Autodesk Inventor part; units mm, degrees
ref_plane "YZ Plane" through (0, 0, 0) normal (1, 0, 0) x (0, 1, 0)
ref_plane "XZ Plane" through (0, 0, 0) normal (0, 1, 0) x (-1, 0, 0)
ref_plane "XY Plane" through (0, 0, 0) normal (0, 0, 1) x (1, 0, 0)
sketch "Skizze1" plane through (0, 0, 0) normal (0, 1, 0) x (-1, 0, 0)
  line L0 (5, 18.5) -> (-5, 18.5)
  line L1 (-5, 18.5) -> (-5, -18.5)
  line L2 (-5, -18.5) -> (5, -18.5)
  line L3 (5, -18.5) -> (5, 18.5)
  line L4 (5, 18.5) -> (-5, -18.5) construction
  line L5 (-5, 18.5) -> (5, -18.5) construction
  circle A0 centre (0, -4.75) radius 13.75 construction
  arc A1 (-5, -17.5587) -> (5, -17.5587) centre (0, -4.75) ccw
  arc A2 (5, 8.0587) -> (-5, 8.0587) centre (0, -4.75) ccw
  line L6 (0, -18.5) -> (0, 9) construction
  circle A3 centre (0, -13.75) radius 1.5
  circle A4 centre (0, 4.25) radius 1.5
  line L7 (-5, -4.75) -> (5, -4.75) construction
  circle A5 centre (0, -13.75) radius 4 construction
  circle A6 centre (0, 4.25) radius 4 construction
  circle A7 centre (0, -4.75) radius 2.75
  point P0 (0, 0)
  point P1 (0, 0)
  dimension "d2" = 37
  dimension "d3" = 10
  dimension "d4" = 27.5
  dimension "d18" = 3
  dimension "d20" = 18
  dimension "d23" = 8
  dimension "d24" = 8
  dimension "d25" = 5.5
extrude "Extrusion1" add sketch "Skizze1" along normal blind 22 contours L3 A2 L1 L0 | L3 A1 L1 A2 | A3 | A4
sketch "Skizze2" plane through (0, 0, 0) normal (1, 0, 0) x (0, 1, 0)
  line L0 (0, -18.5) -> (0, -7.5)
  line L1 (0, 18.5) -> (22, 18.5)
  line L2 (22, -7.5) -> (22, -18.5)
  line L3 (7, -18.5) -> (22, -10.5244)
  line L4 (22, -18.5) -> (0, -18.5)
  line L5 (22, -10.5244) -> (22, -18.5)
  line L6 (22, -18.5) -> (7, -18.5)
  line L7 (0, -7.5) -> (22, -7.5)
  line L8 (22, 18.5) -> (22, -2)
  line L9 (22, -2) -> (0, -2)
  line L10 (0, -2) -> (0, 18.5)
  dimension "d14" = 62
  dimension "d15" = 7
extrude "Extrusion5" cut sketch "Skizze2" along normal through all both and the other way through all contours L3 L2 L4
extrude "Extrusion3" cut sketch "Skizze1" along normal blind 5 contours L3 A1 L1 A2 | L3 L2 A1 | A1 L2 L1 | A3 | A4 | A7
extrude "Extrusion6" cut sketch "Skizze1" along normal blind 11 contours A3 | A4
fillet "Rundung1" radius 1 9 edges at (5, 22, 3.9878) (-5, 22, 3.9878) (0, 22, -10.5244) (5, 15.3852, -14.0415) (5, 6.8852, -17.5587) (-5, 6.8852, -17.5587) (-5, 15.3852, -14.0415) (-5, 11, 18.5) (5, 11, 18.5)
properties part number "Schalter_Knauf"
Input: part model. Units: mm. Frame: model coordinates. A direction names the side the tool comes from. Coordinates: 2 decimals unless noted, no trailing zeros. Loops run counter-clockwise (first coordinate to the right, second up) from the corner with the lowest first, then second, coordinate; pieces in that order, holes last.
Q1. Section B-B, the plane z = 4.25. Return the cut outline in (x, y).
Results are:
outline: (-5, 5) - (-1.5, 5) - (-1.5, 11) - (1.5, 11) - (1.5, 5) - (5, 5) - (5, 21) arc R1 ccw to (4, 22) - (-4, 22) arc R1 ccw to (-5, 21) - close
Q2. Contact query for flat-ended pins moving along their axis: pin 1 (3.5 mm diameter, centred on x = 0, z = -13.75, fed in from -Y); pin 2 (6 mm diameter, centred on x = -3, y = 9, fed in from -Z); pin 3 (1.5 mm diameter, centred on x = -0.5, z = 4.5, fed in from -Y); pin 4 (4.5 mm diameter, centred on x = 0, z = -4.75, fed in from +Y). Output: stop coordinate, or through.
Results are:
pin 1: stops at y = 5
pin 2: stops at z = -18.48
pin 3: stops at y = 11
pin 4: passes through
Q3. Set-up query: faces 1 (the flat face through (0, 11, -14)), 2 (the flat face through (5, 10, 4)), 3 (the cylindrical face through (0, 2, 9)). Return all of +Z, -Z, +X, -X, +Y, -Y with unobstructed straight access to the full face (end or side cutting, diameter ignored); none if empty.
Results are:
face 1: -Y
face 2: +Z, -Z, +X, +Y, -Y
face 3: -Z, -Y
Q4. Section A-A, the plane z = -4.75. Return the cut outline in (x, y), and give its area (3 significant figures).
Results are:
outline: (-5, 5) - (-2.75, 5) - (-2.75, 22) - (-4, 22) arc R1 ccw to (-5, 21) - close; (2.75, 5) - (5, 5) - (5, 21) arc R1 ccw to (4, 22) - (2.75, 22) - close
area: 76.1 mm2
Q5. Section C-C, the plane x = 0.75. Return the cut outline in (y, z), and give its area (3 significant figures).
Results are:
outline: (0, 8.98) - (5, 8.98) - (5, 5.55) - (11, 5.55) - (11, 2.95) - (5, 2.95) - (5, -2.1) - (22, -2.1) - (22, 18.5) - (0, 18.5) - close; (5, -18.48) - (7.04, -18.48) - (21.47, -10.81) arc R1 ccw to (22, -9.92) - (22, -7.4) - (5, -7.4) - (5, -12.45) - (11, -12.45) - (11, -15.05) - (5, -15.05) - close
area: 496 mm2
Q6. Line query: line 1 along Z through (x, y) = (0, 6.45); line 2 along X through (y, z) = (15.25, -4.75); line 3 along X through (y, z) = (9.2, -13.75). Output: solid intervals per line, ascending.
Results are:
line 1: z = -18.5 to -15.25, -12.25 to -7.5, -2 to 2.75, 5.75 to 18.5
line 2: x = -5 to -2.75, 2.75 to 5
line 3: x = -5 to -1.5, 1.5 to 5
Q7. Section D-D, the plane z = 0. Return the cut outline in (x, y).
Results are:
outline: (-5, 5) - (5, 5) - (5, 21) arc R1 ccw to (4, 22) - (-4, 22) arc R1 ccw to (-5, 21) - close
